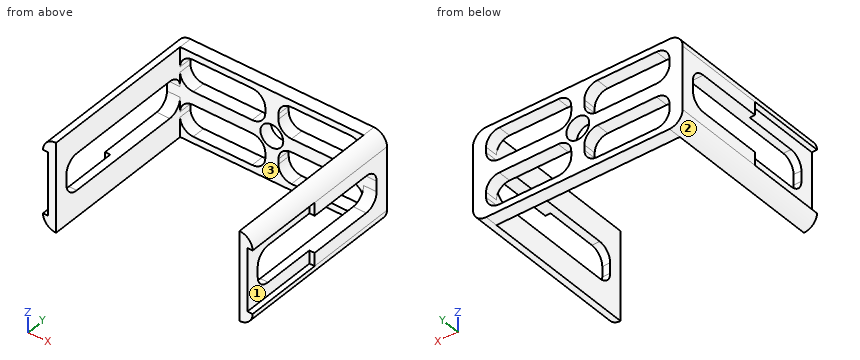
from build123d import *

# Parameters (mm, degrees)
F1_DEPTH  = 10
F2_R      = 8.7132034356
F3_DEPTH  = 11
F4_DEPTH  = 11
F6_DEPTH  = 120
F7_W      = 60
F7_H      = 48
F8_DEPTH  = 4
F10_DEPTH = 10


# Not quite as in the source:
# - a pattern or mirror of a feature is missing from the dataset's text; its kind, count and spacing are read off the source's solid


with BuildPart() as f1:
    # F0 (on Front) → F1 (new body)
    with BuildSketch(Plane.XZ):
        with BuildLine():
            Line((-70, -34), (70, -34))
            ThreePointArc((70, -34), (77.0710678119, -31.0710678119), (80, -24))
            Line((80, -24), (80, 24))
            ThreePointArc((80, 24), (77.0710678119, 31.0710678119), (70, 34))
            Line((70, 34), (-70, 34))
            ThreePointArc((-70, 34), (-77.0710678119, 31.0710678119), (-80, 24))
            Line((-80, 24), (-80, -24))
            ThreePointArc((-80, -24), (-77.0710678119, -31.0710678119), (-70, -34))
        make_face()
    extrude(amount=F1_DEPTH)

    # F2 (on face) → F3 (cut)
    with BuildSketch(Plane.XZ.offset(10)):
        with BuildLine():
            Line((15, 5), (60, 5))
            ThreePointArc((60, 5), (67.0710678119, 7.9289321881), (70, 15))
            Line((70, 15), (70, 19))
            ThreePointArc((70, 19), (67.0710678119, 26.0710678119), (60, 29))
            Line((60, 29), (15, 29))
            ThreePointArc((15, 29), (7.9289321881, 26.0710678119), (5, 19))
            Line((5, 19), (5, 15))
            ThreePointArc((5, 15), (7.9289321881, 7.9289321881), (15, 5))
        make_face()
        with BuildLine():
            ThreePointArc((70, -15), (67.0710678119, -7.9289321881), (60, -5))
            Line((60, -5), (15, -5))
            ThreePointArc((15, -5), (7.9289321881, -7.9289321881), (5, -15))
            Line((5, -15), (5, -19))
            ThreePointArc((5, -19), (7.9289321881, -26.0710678119), (15, -29))
            Line((15, -29), (60, -29))
            ThreePointArc((60, -29), (67.0710678119, -26.0710678119), (70, -19))
            Line((70, -19), (70, -15))
        make_face()
        with BuildLine():
            Line((-15, -5), (-60, -5))
            ThreePointArc((-60, -5), (-67.0710678119, -7.9289321881), (-70, -15))
            Line((-70, -15), (-70, -19))
            ThreePointArc((-70, -19), (-67.0710678119, -26.0710678119), (-60, -29))
            Line((-60, -29), (-15, -29))
            ThreePointArc((-15, -29), (-7.9289321881, -26.0710678119), (-5, -19))
            Line((-5, -19), (-5, -15))
            ThreePointArc((-5, -15), (-7.9289321881, -7.9289321881), (-15, -5))
        make_face()
        with BuildLine():
            ThreePointArc((-5, 19), (-7.9289321881, 26.0710678119), (-15, 29))
            Line((-15, 29), (-60, 29))
            ThreePointArc((-60, 29), (-67.0710678119, 26.0710678119), (-70, 19))
            Line((-70, 19), (-70, 15))
            ThreePointArc((-70, 15), (-67.0710678119, 7.9289321881), (-60, 5))
            Line((-60, 5), (-15, 5))
            ThreePointArc((-15, 5), (-7.9289321881, 7.9289321881), (-5, 15))
            Line((-5, 15), (-5, 19))
        make_face()
        Circle(F2_R)
    extrude(amount=-F3_DEPTH, mode=Mode.SUBTRACT)

    # F2 (on face) → F4 (cut)
    with BuildSketch(Plane.XZ.offset(10)):
        with BuildLine():
            Line((15, 5), (60, 5))
            ThreePointArc((60, 5), (67.0710678119, 7.9289321881), (70, 15))
            Line((70, 15), (70, 19))
            ThreePointArc((70, 19), (67.0710678119, 26.0710678119), (60, 29))
            Line((60, 29), (15, 29))
            ThreePointArc((15, 29), (7.9289321881, 26.0710678119), (5, 19))
            Line((5, 19), (5, 15))
            ThreePointArc((5, 15), (7.9289321881, 7.9289321881), (15, 5))
        make_face()
        with BuildLine():
            ThreePointArc((70, -15), (67.0710678119, -7.9289321881), (60, -5))
            Line((60, -5), (15, -5))
            ThreePointArc((15, -5), (7.9289321881, -7.9289321881), (5, -15))
            Line((5, -15), (5, -19))
            ThreePointArc((5, -19), (7.9289321881, -26.0710678119), (15, -29))
            Line((15, -29), (60, -29))
            ThreePointArc((60, -29), (67.0710678119, -26.0710678119), (70, -19))
            Line((70, -19), (70, -15))
        make_face()
        with BuildLine():
            Line((-15, -5), (-60, -5))
            ThreePointArc((-60, -5), (-67.0710678119, -7.9289321881), (-70, -15))
            Line((-70, -15), (-70, -19))
            ThreePointArc((-70, -19), (-67.0710678119, -26.0710678119), (-60, -29))
            Line((-60, -29), (-15, -29))
            ThreePointArc((-15, -29), (-7.9289321881, -26.0710678119), (-5, -19))
            Line((-5, -19), (-5, -15))
            ThreePointArc((-5, -15), (-7.9289321881, -7.9289321881), (-15, -5))
        make_face()
        with BuildLine():
            ThreePointArc((-5, 19), (-7.9289321881, 26.0710678119), (-15, 29))
            Line((-15, 29), (-60, 29))
            ThreePointArc((-60, 29), (-67.0710678119, 26.0710678119), (-70, 19))
            Line((-70, 19), (-70, 15))
            ThreePointArc((-70, 15), (-67.0710678119, 7.9289321881), (-60, 5))
            Line((-60, 5), (-15, 5))
            ThreePointArc((-15, 5), (-7.9289321881, 7.9289321881), (-5, 15))
            Line((-5, 15), (-5, 19))
        make_face()
        Circle(F2_R)
    extrude(amount=-F4_DEPTH, mode=Mode.SUBTRACT)

    # F5 (on face) → F6 (join)
    with BuildSketch(Plane.XZ.offset(10)):
        with BuildLine():
            Line((70, 34), (70, -34))
            ThreePointArc((70, -34), (77.0710678119, -31.0710678119), (80, -24))
            Line((80, -24), (80, 24))
            ThreePointArc((80, 24), (77.0710678119, 31.0710678119), (70, 34))
        make_face()
        with BuildLine():
            ThreePointArc((-80, -24), (-77.0710678119, -31.0710678119), (-70, -34))
            Line((-70, -34), (-70, 34))
            ThreePointArc((-70, 34), (-77.0710678119, 31.0710678119), (-80, 24))
            Line((-80, 24), (-80, -24))
        make_face()
    extrude(amount=F6_DEPTH)

    # F7 (on face) → F8 (cut)
    with BuildSketch(Plane(origin=(-80, 0, 0), x_dir=(0, -1, 0), z_dir=(-1, 0, 0))):
        with Locations((100, 0)):
            Rectangle(F7_W, F7_H)
    f8 = extrude(amount=-F8_DEPTH, mode=Mode.SUBTRACT)

    # F8_copies: F8 across plane
    add(f8.mirror(Plane(origin=(0, 0, 0), x_dir=(0, 0, 1), z_dir=(1, 0, 0))), mode=Mode.SUBTRACT)

    # F9 (on face) → F10 (cut)
    with BuildSketch(Plane(origin=(-80, 0, 0), x_dir=(0, -1, 0), z_dir=(-1, 0, 0))):
        with BuildLine():
            Line((20, -14), (110, -14))
            ThreePointArc((110, -14), (117.0710678119, -11.0710678119), (120, -4))
            Line((120, -4), (120, 4))
            ThreePointArc((120, 4), (117.0710678119, 11.0710678119), (110, 14))
            Line((110, 14), (20, 14))
            ThreePointArc((20, 14), (12.9289321881, 11.0710678119), (10, 4))
            Line((10, 4), (10, -4))
            ThreePointArc((10, -4), (12.9289321881, -11.0710678119), (20, -14))
        make_face()
    f10 = extrude(amount=-F10_DEPTH, mode=Mode.SUBTRACT)

    # F10_copies: F10 across plane
    add(f10.mirror(Plane(origin=(0, 0, 0), x_dir=(0, 0, 1), z_dir=(1, 0, 0))), mode=Mode.SUBTRACT)


solid = f1.part
Geometry check sheet. Reference: the model listing, model coordinates, mm. Face numbers are marked on the shaded views. Give positions to 0.01 mm unless a question says otherwise; leave off trailing zeros. Order: outer loops, then holes, each group sorted by start corner. A loop starts at its lowest first (then second) coordinate and runs counter-clockwise, first axis right, second up.
1) Cross-section at B-B (x = -19). Record the boundary of the cut face in (y, z), then the cut area to 3 significant figures.
Results are:
outline: (-10, -34) - (0, -34) - (0, -29) - (-10, -29) - close; (-10, -5) - (0, -5) - (0, 5) - (-10, 5) - close; (-10, 29) - (0, 29) - (0, 34) - (-10, 34) - close
area: 200 mm2
2) Cross-section at D-D (y = -94.5). Record the boundary of the cut face in (x, z), then the cut area to 3 significant figures.
Results are:
outline: (-80, -24) arc R10 ccw to (-70, -34) - (-70, -14) - (-76, -14) - (-76, -24) - close; (-80, 24) - (-76, 24) - (-76, 14) - (-70, 14) - (-70, 34) arc R10 ccw to start; (70, -34) arc R10 ccw to (80, -24) - (76, -24) - (76, -14) - (70, -14) - close; (70, 14) - (76, 14) - (76, 24) - (80, 24) arc R10 ccw to (70, 34) - close
area: 554 mm2
3) Draft check along X on the marked faces 1, 2 and 3. Enter one of: released by +X, released by -X, zero draft, split by the parting line, or undercut.
Results are:
face 1: released by +X
face 2: released by -X
face 3: undercut
4) Cross-section at C-C (z = 0). Record the boundary of the cut face in (x, y), then the cut area to 3 significant figures.
Results are:
outline: (-80, -10) - (-8.71, -10) - (-8.71, 0) - (-80, 0) - close; (-76, -130) - (-70, -130) - (-70, -120) - (-76, -120) - close; (8.71, -10) - (80, -10) - (80, 0) - (8.71, 0) - close; (70, -130) - (76, -130) - (76, -120) - (70, -120) - close
area: 1,550 mm2
5) Cross-section at A-A (x = 0). Record the boundary of the cut face in (y, z), then the cut area to 3 significant figures.
Results are:
outline: (-10, -34) - (0, -34) - (0, -8.71) - (-10, -8.71) - close; (-10, 8.71) - (0, 8.71) - (0, 34) - (-10, 34) - close
area: 506 mm2
6) Gauge pin test, flat ends, axial feed: pin 1 (4.5 mm diameter, centred on x = -78.5, z = 21, fed in from -Y); pin 2 (8 mm diameter, centred on y = -87, z = -13.5, fed in from -X); pin 3 (24 mm diameter, centred on y = -95, z = 9, fed in from +X); pin 4 (6 mm diameter, centred on x = 12, z = 22.5, fed in from -Y). Record the tip position at first contact, or that the pin passes through.
Results are:
pin 1: stops at y = -70
pin 2: stops at x = -76
pin 3: stops at x = 76
pin 4: passes through
7) Material ranges on probe 1 along Z at (x, y) = (0, -7); probe 2 along X at (y, z) = (-102.5, -20); probe 3 along Y at (x, z) = (73.5, 5), recorded low to high.
Results are:
probe 1: z = -34 to -8.71, 8.71 to 34
probe 2: x = -76 to -70, 70 to 76
probe 3: y = -130 to -119.95, -10.05 to 0
